from build123d import *

# Parameters (mm, degrees)
EXTRUDE_1_DEPTH              = 5
EXTRUDE_2_DEPTH              = 15
HOLE_WIZARD_M2_1_D           = 2.35
HOLE_WIZARD_M2_1_DEPTH       = 20
HOLE_WIZARD_M2_1_CBORE_D     = 4.35
HOLE_WIZARD_M2_1_CBORE_DEPTH = 3


with BuildPart() as part:
    # 草圖1 → 填料-伸長1 (new body)
    with BuildSketch(Plane.XZ.offset(5)):
        Polygon((3.4, 1.962990915), (0, 0), (0, -3.92598183), (19.084609691, -14.944486373), (22.484609691, -9.055513627), align=None)
    extrude(amount=-EXTRUDE_1_DEPTH)

    # 草圖2 → 填料-伸長2 (add)
    with BuildSketch(Plane.XZ.offset(5)):
        Polygon((3, 1.732050808), (3, -2.997949192), (0, -2.997949192), (0, 0), align=None)
    extrude(amount=EXTRUDE_2_DEPTH)

    # M2 六角頭機械螺釘的柱孔1
    with Locations(Plane(origin=(0, 0, 0), x_dir=(1, 0, 0), z_dir=(0, 1, 0))):
        with Locations((17.926725858, 10.35), (10.998522628, 6.35)):
            CounterBoreHole(HOLE_WIZARD_M2_1_D / 2, HOLE_WIZARD_M2_1_CBORE_D / 2, HOLE_WIZARD_M2_1_CBORE_DEPTH, depth=HOLE_WIZARD_M2_1_DEPTH)


solid = part.part
Build history of the part. All positions in model axes, mm. A direction names the side the tool comes from. Give positions to 0.01 mm unless a question says otherwise; leave off trailing zeros. Order: outer loops, then holes, each group sorted by start corner. A loop starts at its lowest first (then second) coordinate and runs counter-clockwise, first axis right, second up. Notation, with made-up numbers: M 42,30.25 L 86,30.25 A23 ccw 86,60.25 Z; hole C 28.5,65.25 d11. An arc over 180 degrees is marked long. Use one line per item in the form item = value.
1) Saw through at A-A (y = -3.5). Give the cut face in (x, z) (3 decimals), plus the area to 3 significant figures.
Calculated:
outline = M 0,-3.926 L 19.085,-14.944 L 22.485,-9.056 L 3.4,1.963 L 0,0 Z; hole C 10.999,-6.35 d2.35; hole C 17.927,-10.35 d2.35
area = 148 mm2
2) Drop flat-ended pins along their axis: pin 1 (6 mm diameter, centred on x = 10, y = -4.5, fed in from +Z); pin 2 (5 mm diameter, centred on x = 13, z = -9, fed in from -Y); pin 3 (2 mm diameter, centred on x = 20, y = -5, fed in from -Z); pin 4 (6 mm diameter, centred on y = -2.5, z = -12, fed in from -X). Give the stop position or say it passes through.
Calculated:
pin_1 = -0.12
pin_2 = -5
pin_3 = -14.94
pin_4 = 8.79
3) Tool access for faces 4 (the face through (12, -1.48, -4.42)), 5 (the face through (3, -12, -1)), 6 (the face through (2, -12, -2.998)), 7 (the face through (0, -10, -2)), 8 (the face through (9.41, -2.54, -9.36)): list every direction of +Z, -Z, +X, -X, +Y, -Y with a clear straight run to the whole face (end or side of a thin tool).
Calculated:
face_4 = +Y
face_5 = +Z, -Z, +X, -Y
face_6 = -Z, +X, -X, -Y
face_7 = +Z, -Z, -X, +Y, -Y
face_8 = -Z, -X, +Y, -Y
4) Two-plate mould, pull along X, no slides. Class faces 1 (the face through (11, -5, -4)), 2 (the face through (20.76, -2.54, -12.04)), 3 (the face through (12, -3, -5)): released by +X, released by -X, zero draft, split by the parting line, or undercut.
Calculated:
face_1 = zero draft
face_2 = released by +X
face_3 = undercut
5) Saw through at D-D (z = 1). Give the cut face in (x, y), plus the area to 3 significant figures.
Calculated:
outline = M 1.73,-20 L 3,-20 L 3,-5 L 5.07,-5 L 5.07,0 L 1.73,0 Z
area = 35.7 mm2
6) Saw through at B-B (z = -6.35). Give the cut face in (x, y), plus the area to 4 significant figures.
Calculated:
outline = M 4.2,-5 L 9.82,-5 L 9.82,-3 L 8.82,-3 L 8.82,0 L 4.2,0 Z; M 12.17,-5 L 17.8,-5 L 17.8,0 L 13.17,0 L 13.17,-3 L 12.17,-3 Z
area = 50.25 mm2
7) Saw through at C-C (x = 10.25). Give the cut face in (y, z), plus the area to 3 significant figures.
Calculated:
outline = M -5,-9.84 L 0,-9.84 L 0,-8.39 L -3,-8.39 L -3,-7.26 L -5,-7.26 Z; M -5,-5.44 L -3,-5.44 L -3,-4.31 L 0,-4.31 L 0,-1.99 L -5,-1.99 Z
area = 23.4 mm2
8) Probe probe 1 along Y at (x, z) = (13.75, -5.25); probe 2 along Y at (x, z) = (9.5, -6.75); probe 3 along X at (y, z) = (-4.05, -10.35). List the from-to ranges inside material, lowest first.
Calculated:
probe_1 = -5 to 0
probe_2 = -5 to -3
probe_3 = 11.13 to 16.75, 19.1 to 21.74
